from build123d import *

# Parameters (mm, degrees)
EXTRUDE_1_DEPTH     = 4
SKETCH_2_R          = 1.5
EXTRUDE_2_DEPTH     = 4
SKETCH_3_R          = 1.5
CUT_EXTRUDE_1_DEPTH = 4
FILLET_1_R          = 10
SKETCH_4_R          = 0.5
CUT_EXTRUDE_2_DEPTH = 4


with BuildPart() as part:
    # 草图1 → 凸台-拉伸1 (new body)
    with BuildSketch(Plane.XY):
        Polygon((-5.5, 0), (-11.5, 0), (-11.5, 24.03), (-20.5, 15.03), (-20.5, 0), (-45, 0), (-45, 5), (-5, 30), (0, 30), (0, 25), (-5.5, 25), align=None)
    extrude(amount=EXTRUDE_1_DEPTH)

    # 草图2 → 凸台-拉伸2 (add)
    with BuildSketch(Plane.XY.offset(4)):
        with BuildLine():
            Line((-6.5, 30), (-5, 30))
            Line((-5, 30), (-12.5, 25.3125))
            Line((-12.5, 25.3125), (-12.5, 30))
            ThreePointArc((-12.5, 30), (-9.5, 33), (-6.5, 30))
        make_face()
        with Locations((-9.5, 30)):
            Circle(SKETCH_2_R, mode=Mode.SUBTRACT)
    extrude(amount=-EXTRUDE_2_DEPTH)

    # 草图3 → 切除-拉伸1 (cut)
    with BuildSketch(Plane.XY.offset(4)):
        with Locations((-30.810217499, 10.330871139)):
            Circle(SKETCH_3_R)
    extrude(amount=-CUT_EXTRUDE_1_DEPTH, mode=Mode.SUBTRACT)

    # 圆角1
    fillet_1_edges = [part.edges().sort_by_distance(p)[0] for p in [
        (-6.5, 30, 2),
        (-12.5, 25.3125, 2),
    ]]
    fillet(fillet_1_edges, radius=FILLET_1_R)

    # 草图4 → 切除-拉伸2 (cut)
    with BuildSketch(Plane.XY.offset(4)):
        with Locations((-5.5, 25)):
            Circle(SKETCH_4_R)
        with Locations((-11.5, 24.03)):
            Circle(SKETCH_4_R)
        with Locations((-20.5, 15.03)):
            Circle(SKETCH_4_R)
    extrude(amount=-CUT_EXTRUDE_2_DEPTH, mode=Mode.SUBTRACT)


solid = part.part
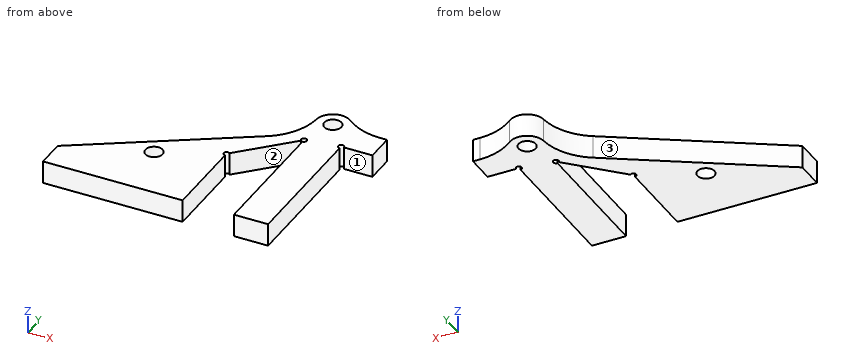
Source: CAD feature listing. Evaluate the final solid. Frame: model axes, mm. Face numbers are marked on the shaded views. Coordinates: 2 decimals unless noted, no trailing zeros. Order: outer loops, then holes, each group sorted by start corner. A loop starts at its lowest first (then second) coordinate and runs counter-clockwise, first axis right, second up.
Item 1: Cut plane B-B (x = -30.5). Return loops of the section in (y, z), plus the area to 3 significant figures.
Output values:
outline: (0, 0) - (8.86, 0) - (8.86, 4) - (0, 4) - close; (11.8, 0) - (14.06, 0) - (14.06, 4) - (11.8, 4) - close
area: 44.5 mm2
Item 2: Pull-direction query (X, two-part tool) for the marked faces 1, 2 and 3; classes: pulls with the +X half, pulls with the -X half, needs draft (parallel to the pull), parting line crosses it, or undercut.
Output values:
face 1: needs draft
face 2: undercut
face 3: pulls with the -X half
Item 3: Material intervals for line 1 (X direction, y = 9.5, z = 0.75); line 2 (X direction, y = 22.5, z = 3.55); line 3 (X direction, y = 15.03, z = 1.6), sorted ascending.
Output values:
line 1: x = -37.8 to -32.06, -29.56 to -20.5, -11.5 to -5.5
line 2: x = -17 to -13.03, -11.5 to -5.5
line 3: x = -28.95 to -21, -11.5 to -5.5
Item 4: First-contact query: P1, Ø2, axis at x = -2.5, z = 2, coming from the -Y side; P2, Ø2.5, axis at x = -9.5, y = 30, coming from the +Z side; P3, Ø2, axis at y = 18.5, z = 1.5, coming from the +X side; P4, Ø2, axis at y = 15.5, z = 1.5, coming from the -X side. Flat tips, straight axial feed; report the tip coordinate or a pass-through.
Output values:
P1: stops at y = 25
P2: passes through
P3: stops at x = -5.5
P4: stops at x = -29.8
Item 5: Cut plane D-D (x = -21.5). Return loops of the section in (y, z), plus the area to 4 significant figures.
Output values:
outline: (0, 0) - (19.69, 0) - (19.69, 4) - (0, 4) - close
area: 78.75 mm2
Item 6: Cut plane C-C (z = 2.3). Count the separate pieces of the cut face and the enclosed holes in it, plus the area to 3 significant figures.
Output values:
separate pieces: 1
enclosed holes: 2
area: 560 mm2
Item 7: Cut plane A-A (y = 13.5). Return loops of the section in (x, z).
Output values:
outline: (-31.4, 0) - (-20.5, 0) - (-20.5, 4) - (-31.4, 4) - close; (-11.5, 0) - (-5.5, 0) - (-5.5, 4) - (-11.5, 4) - close
